Here's the drawing with two shaded views (mm, measured from the low corner). I have some questions. Give positions to 0.01 mm unless a question says otherwise; leave off trailing zeros. Write each loop counter-clockwise with the first axis right and the second up, starting at its lowest first coordinate (ties: lowest second). Pieces come first, ordered by that corner, then holes. Notation, with made-up numbers: (-19.75, -6) - (3.25, -6) arc R18 ccw to (3.25, 6) - close; hole circle Ø2 at (54.5, 75). An arc over 180 degrees is marked (long way). Write item = value, one per line.
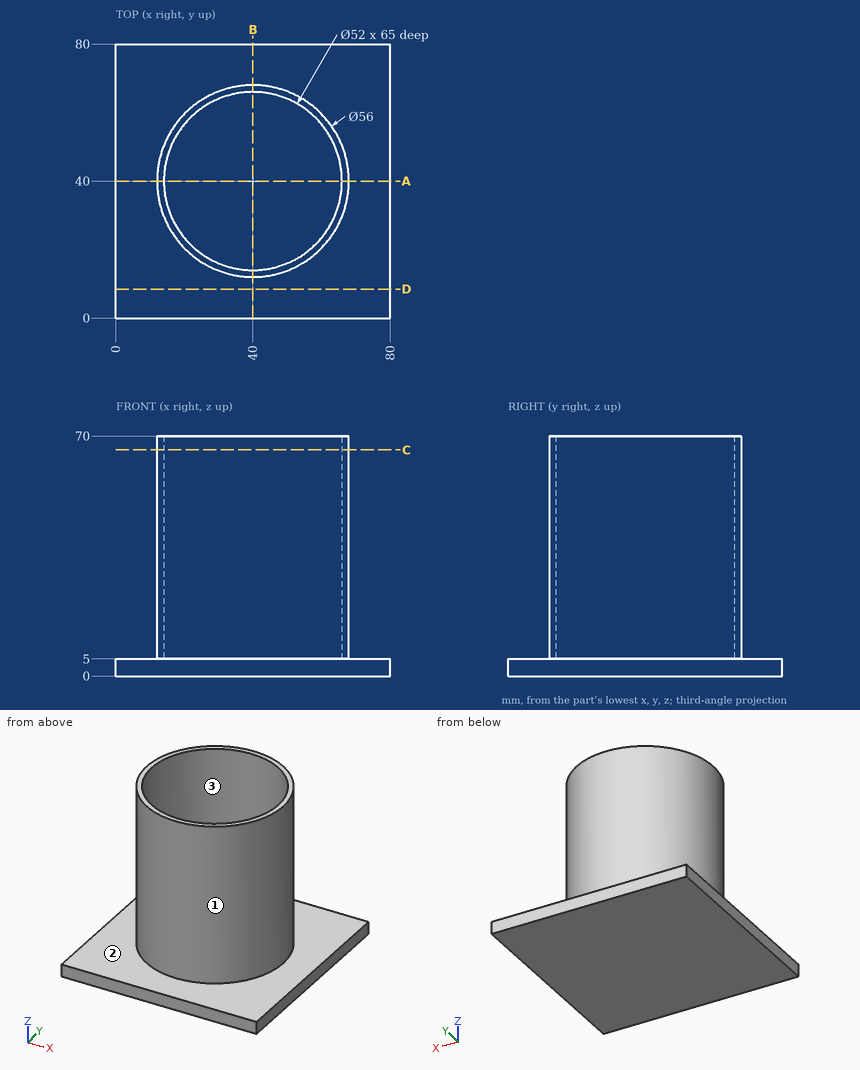
1. I need wall thicknesses on line 1 (Y direction, x = 40, z = 33); line 2 (Z direction, x = 45.5, y = 35); line 3 (Y direction, x = 43.5, z = 24). Which ranges of each line are inside material? Lowest first, please.
Filled sheet:
line_1 = 12 to 14, 66 to 68
line_2 = 0 to 5
line_3 = 12.22 to 14.24, 65.76 to 67.78
2. If we section it at D-D, the plane y = 8.5: Please give me the cut outline in (x, z).
Filled sheet:
outline = (0, 0) - (80, 0) - (80, 5) - (0, 5) - close
3. If we section it at A-A, the plane y = 40: Please give me the cut outline in (x, z), and give its area (3 significant figures).
Filled sheet:
outline = (0, 0) - (80, 0) - (80, 5) - (68, 5) - (68, 70) - (66, 70) - (66, 5) - (14, 5) - (14, 70) - (12, 70) - (12, 5) - (0, 5) - close
area = 660 mm2
4. If we section it at C-C, the plane z = 66: Please give me the cut outline in (x, y), and give its area (3 significant figures).
Filled sheet:
outline = circle Ø56 at (40, 40); hole circle Ø52 at (40, 40)
area = 339 mm2
5. Thinking about a two-plate mould opening in Y: for the marked faces 1, 2 and 3, which applies, pulls with the +Y half, pulls with the -Y half, needs draft (parallel to the pull), parting line crosses it, or undercut?
Filled sheet:
face_1 = parting line crosses it
face_2 = needs draft
face_3 = undercut
6. For pin 1 (8 mm diameter, centred on y = 60, z = 34.5, fed in from +X); pin 2 (10 mm diameter, centred on x = 66, y = 50, fed in from -Z); pin 3 (6 mm diameter, centred on y = 23.5, z = 41, fed in from -X); pin 4 (10 mm diameter, centred on y = 22.5, z = 57, fed in from +X), each with a flat end and sliding along its axis, tell me the tip position at first contact or that it passes through.
Filled sheet:
pin_1 = 62.98
pin_2 = 0
pin_3 = 15.47
pin_4 = 65.05
